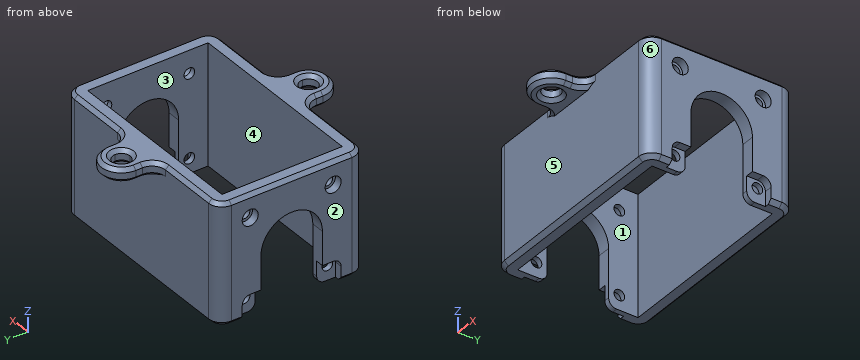
```python
from build123d import *

# Parameters (mm, degrees)
F0_W          = 70
F0_H          = 45
F1_DEPTH      = 45
F2_R          = 2
F3_DEPTH      = 40.001
F3_DEPTH_BACK = 40.001
F5_R          = 3
F6_DEPTH      = 3
F7_R          = 3
F8_DEPTH      = 3
F9_R          = 3
F10_SIZE      = 1.5
F12_DEPTH     = 5
F13_R         = 5
F14_T1_DEPTH  = 22.5
F14_T3_DEPTH  = 22.5
F14_T5_DEPTH  = 2.5
F14_T7_DEPTH  = 45
F14_T9_DEPTH  = 2.5
F14_T16_ANGLE = 180
F14_T22_ANGLE = 128.3255006626
F14_T27_ANGLE = 90
F14_T29_ANGLE = 90
F14_T31_ANGLE = 180
F14_T33_ANGLE = 90
F14_T35_ANGLE = 90
F14_T37_ANGLE = 90
F14_T39_ANGLE = 90
F14_T41_ANGLE = 180
F14_T43_ANGLE = 90
F14_T45_ANGLE = 90
F14_T49_ANGLE = 128.3255006626
F14_T52_ANGLE = 180
F14_T56_ANGLE = 128.3255006626
F14_T61_ANGLE = 128.3255006626


# Not quite as in the source:
# - a fillet or chamfer that OpenCascade refuses, or shapes differently, is made with other operations: its cross-section is extruded or revolved along the edge and cut away or added


with BuildPart() as f1:
    # F0 (on Top) → F1 (new body)
    with BuildSketch(Plane.XY):
        with BuildLine():
            ThreePointArc((40, 22.5), (38.5355339059, 26.0355339059), (35, 27.5))
            Line((35, 27.5), (-35, 27.5))
            ThreePointArc((-35, 27.5), (-38.5355339059, 26.0355339059), (-40, 22.5))
            Line((-40, 22.5), (-40, -22.5))
            ThreePointArc((-40, -22.5), (-38.5355339059, -26.0355339059), (-35, -27.5))
            Line((-35, -27.5), (35, -27.5))
            ThreePointArc((35, -27.5), (38.5355339059, -26.0355339059), (40, -22.5))
            Line((40, -22.5), (40, 22.5))
        make_face()
        Rectangle(F0_W, F0_H, mode=Mode.SUBTRACT)
    extrude(amount=F1_DEPTH)

    # F2 (on Right) → F3 (cut, two sides)
    with BuildSketch(Plane.YZ) as f3_sk:
        with Locations((15.5, 36.5)):
            Circle(F2_R)
        with Locations((-15.5, 36.5)):
            Circle(F2_R)
        with Locations((15.5, 5.5)):
            Circle(F2_R)
        with Locations((-15.5, 5.5)):
            Circle(F2_R)
        with BuildLine():
            Line((11.5, 0), (11.5, 21))
            ThreePointArc((11.5, 21), (0, 32.5), (-11.5, 21))
            Line((-11.5, 21), (-11.5, 0))
            Line((-11.5, 0), (11.5, 0))
        make_face()
    extrude(amount=-F3_DEPTH, mode=Mode.SUBTRACT)
    extrude(f3_sk.sketch, amount=F3_DEPTH_BACK, mode=Mode.SUBTRACT)

    # F5 (on face) → F6 (cut)
    with BuildSketch(Plane.YZ.offset(40)):
        with Locations((-15.5, 36.5)):
            Circle(F5_R)
        with Locations((15.5, 36.5)):
            Circle(F5_R)
        with BuildLine():
            ThreePointArc((-15.5, 8.5), (-17.6213203436, 7.6213203436), (-18.5, 5.5))
            Line((-18.5, 5.5), (-18.5, 0))
            Line((-18.5, 0), (-11.5, 0))
            Line((-11.5, 0), (-11.5, 8.5))
            Line((-11.5, 8.5), (-15.5, 8.5))
        make_face()
        with BuildLine():
            Line((15.5, 8.5), (11.5, 8.5))
            Line((11.5, 8.5), (11.5, 0))
            Line((11.5, 0), (18.5, 0))
            Line((18.5, 0), (18.5, 5.5))
            ThreePointArc((18.5, 5.5), (17.6213203436, 7.6213203436), (15.5, 8.5))
        make_face()
    extrude(amount=-F6_DEPTH, mode=Mode.SUBTRACT)

    # F7 (on face) → F8 (cut)
    with BuildSketch(Plane(origin=(-40, 0, 0), x_dir=(0, -1, 0), z_dir=(-1, 0, 0))):
        with Locations((-15.5, 36.5)):
            Circle(F7_R)
        with Locations((15.5, 36.5)):
            Circle(F7_R)
        with BuildLine():
            Line((11.5, 0), (18.5, 0))
            Line((18.5, 0), (18.5, 5.5))
            ThreePointArc((18.5, 5.5), (17.6213203436, 7.6213203436), (15.5, 8.5))
            Line((15.5, 8.5), (11.5, 8.5))
            Line((11.5, 8.5), (11.5, 0))
        make_face()
        with BuildLine():
            Line((-11.5, 8.5), (-15.5, 8.5))
            ThreePointArc((-15.5, 8.5), (-17.6213203436, 7.6213203436), (-18.5, 5.5))
            Line((-18.5, 5.5), (-18.5, 0))
            Line((-18.5, 0), (-11.5, 0))
            Line((-11.5, 0), (-11.5, 8.5))
        make_face()
    extrude(amount=-F8_DEPTH, mode=Mode.SUBTRACT)

    # F9
    f9_edges = [f1.edges().sort_by_distance(p)[0] for p in [
        (36, 11.5, 0),
        (-36, 11.5, 0),
        (-36, -11.5, 0),
        (36, -11.5, 0),
    ]]
    fillet(f9_edges, radius=F9_R)

    # F10
    f10_edges = [f1.edges().sort_by_distance(p)[0] for p in [
        (-40, 20.5, 0),
        (-38.535534, -26.035534, 0),
        (-40, -20.5, 0),
        (0, -27.5, 0),
        (38.535534, -26.035534, 0),
        (40, -20.5, 0),
        (40, 20.5, 0),
        (38.535534, 26.035534, 0),
        (0, 27.5, 0),
        (-38.535534, 26.035534, 0),
    ]]
    chamfer(f10_edges, length=F10_SIZE)

    # F11 (on face) → F12 (join)
    with BuildSketch(Plane.XY.offset(45)):
        with BuildLine():
            Line((-7.5, 27.5), (0, 27.5))
            Line((0, 27.5), (7.5, 27.5))
            Line((7.5, 27.5), (7.5, 35))
            ThreePointArc((7.5, 35), (0, 42.5), (-7.5, 35))
            Line((-7.5, 35), (-7.5, 27.5))
        make_face()
        with BuildLine():
            ThreePointArc((0, 31.75), (-2.2980970389, 37.2980970389), (3.25, 35))
            ThreePointArc((3.25, 35), (2.2980970389, 32.7019029611), (0, 31.75))
        make_face(mode=Mode.SUBTRACT)
        with BuildLine():
            Line((7.5, -22.5), (0, -22.5))
            Line((0, -22.5), (-7.5, -22.5))
            Line((-7.5, -22.5), (-7.5, -35))
            ThreePointArc((-7.5, -35), (0, -42.5), (7.5, -35))
            Line((7.5, -35), (7.5, -22.5))
        make_face()
        with BuildLine():
            ThreePointArc((3.25, -35), (-2.2980970389, -37.2980970389), (0, -31.75))
            ThreePointArc((0, -31.75), (2.2980970389, -32.7019029611), (3.25, -35))
        make_face(mode=Mode.SUBTRACT)
    extrude(amount=-F12_DEPTH)

    # F13
    f13_edges = [f1.edges().sort_by_distance(p)[0] for p in [
        (7.5, 27.5, 42.5),
        (-7.5, 27.5, 42.5),
        (-7.5, -27.5, 42.5),
        (7.5, -27.5, 42.5),
    ]]
    fillet(f13_edges, radius=F13_R)

    # F14: chamfer of 1.3 on 34 edges, made by hand

    # F14_s2 → F14_t1 (cut)
    with BuildSketch(Plane.YZ.offset(12.5)):
        Polygon((-27.5, 43.7), (-26.2, 45), (-27.5, 45), align=None)
        Polygon((26.2, 45), (27.5, 43.7), (27.5, 45), align=None)
    extrude(amount=F14_T1_DEPTH, mode=Mode.SUBTRACT)

    # F14_s4 → F14_t3 (cut)
    with BuildSketch(Plane.YZ.offset(-35)):
        Polygon((-27.5, 43.7), (-26.2, 45), (-27.5, 45), align=None)
        Polygon((26.2, 45), (27.5, 43.7), (27.5, 45), align=None)
    extrude(amount=F14_T3_DEPTH, mode=Mode.SUBTRACT)

    # F14_s6 → F14_t5 (cut)
    with BuildSketch(Plane.XZ.offset(32.5)):
        Polygon((6.2, 45), (7.5, 43.7), (7.5, 45), align=None)
        Polygon((-6.2, 45), (-7.5, 43.7), (-7.5, 45), align=None)
        Polygon((-6.2, 40), (-7.5, 41.3), (-7.5, 40), align=None)
        Polygon((6.2, 40), (7.5, 41.3), (7.5, 40), align=None)
    extrude(amount=F14_T5_DEPTH, mode=Mode.SUBTRACT)

    # F14_s8 → F14_t7 (cut)
    with BuildSketch(Plane.XZ.offset(-22.5)):
        Polygon((38.7, 45), (40, 43.7), (40, 45), align=None)
        Polygon((-38.7, 45), (-40, 43.7), (-40, 45), align=None)
    extrude(amount=F14_T7_DEPTH, mode=Mode.SUBTRACT)

    # F14_s10 → F14_t9 (cut)
    with BuildSketch(Plane.XZ.offset(-35)):
        Polygon((6.2, 45), (7.5, 43.7), (7.5, 45), align=None)
        Polygon((-6.2, 45), (-7.5, 43.7), (-7.5, 45), align=None)
        Polygon((7.5, 41.3), (6.2, 40), (7.5, 40), align=None)
        Polygon((-7.5, 41.3), (-6.2, 40), (-7.5, 40), align=None)
    extrude(amount=F14_T9_DEPTH, mode=Mode.SUBTRACT)

    # F14_s11 → F14_t12 (revolve, cut)
    with BuildSketch(Plane.XZ.offset(35)):
        Polygon((4.55, 45), (3.25, 43.7), (3.25, 45), align=None)
    revolve(axis=Axis((0, -35, 45), (0, 0, -1)), mode=Mode.SUBTRACT)

    # F14_s13 → F14_t14 (revolve, cut)
    with BuildSketch(Plane.XZ.offset(-35)):
        Polygon((4.55, 45), (3.25, 43.7), (3.25, 45), align=None)
    revolve(axis=Axis((0, 35, 45), (0, 0, -1)), mode=Mode.SUBTRACT)

    # F14_s15 → F14_t16 (revolve, cut)
    with BuildSketch(Plane.XZ.offset(-35)):
        Polygon((7.5, 41.3), (6.2, 40), (7.5, 40), align=None)
    revolve(axis=Axis((0, 35, 40), (0, 0, 1)), revolution_arc=F14_T16_ANGLE, mode=Mode.SUBTRACT)

    # F14_s17 → F14_t18 (revolve, cut)
    with BuildSketch(Plane.XZ.offset(-35)):
        Polygon((3.25, 41.3), (4.55, 40), (3.25, 40), align=None)
    revolve(axis=Axis((0, 35, 40), (0, 0, -1)), mode=Mode.SUBTRACT)


with BuildPart() as f14_tool20:
    # F14_s21 → F14_t22 (revolve)
    with BuildSketch(Plane(origin=(-23.5039658434, -18.5793051911, 0), x_dir=(0, 0, 1), z_dir=(-0.7845004474, -0.6201282512, 0))):
        Polygon((40, -11.4446614013), (41.3, -12.7446614013), (40, -12.7446614013), align=None)
    revolve(axis=Axis((-12.5, -32.5, 40), (0, 0, -1)), revolution_arc=F14_T22_ANGLE)

    split(bisect_by=Plane.XZ.offset(27.5), keep=Keep.TOP)


with BuildPart() as f1_1:
    add(f1.part)

    # F14_t19: cut F14_tool20
    add(f14_tool20.part, mode=Mode.SUBTRACT)

    # F14_s24 → F14_t25 (revolve, cut)
    with BuildSketch(Plane.XZ.offset(35)):
        Polygon((4.55, 40), (3.25, 41.3), (3.25, 40), align=None)
    revolve(axis=Axis((0, -35, 40), (0, 0, -1)), mode=Mode.SUBTRACT)

    # F14_s26 → F14_t27 (revolve, cut)
    with BuildSketch(Plane.YZ.offset(12.5)):
        Polygon((-26.2, 45), (-27.5, 43.7), (-27.5, 45), align=None)
    revolve(axis=Axis((12.5, -32.5, 45), (0, 0, 1)), revolution_arc=F14_T27_ANGLE, mode=Mode.SUBTRACT)

    # F14_s28 → F14_t29 (revolve, cut)
    with BuildSketch(Plane.YZ.offset(35)):
        Polygon((-26.2, 45), (-27.5, 43.7), (-27.5, 45), align=None)
    revolve(axis=Axis((35, -22.5, 45), (0, 0, 1)), revolution_arc=F14_T29_ANGLE, mode=Mode.SUBTRACT)

    # F14_s30 → F14_t31 (revolve, cut)
    with BuildSketch(Plane.XZ.offset(35)):
        Polygon((-6.2, 45), (-7.5, 43.7), (-7.5, 45), align=None)
    revolve(axis=Axis((0, -35, 45), (0, 0, 1)), revolution_arc=F14_T31_ANGLE, mode=Mode.SUBTRACT)

    # F14_s32 → F14_t33 (revolve, cut)
    with BuildSketch(Plane.XZ.offset(-22.5)):
        Polygon((38.7, 45), (40, 43.7), (40, 45), align=None)
    revolve(axis=Axis((35, 22.5, 45), (0, 0, 1)), revolution_arc=F14_T33_ANGLE, mode=Mode.SUBTRACT)

    # F14_s34 → F14_t35 (revolve, cut)
    with BuildSketch(Plane.YZ.offset(-12.5)):
        Polygon((-26.2, 45), (-27.5, 43.7), (-27.5, 45), align=None)
    revolve(axis=Axis((-12.5, -32.5, 45), (0, 0, -1)), revolution_arc=F14_T35_ANGLE, mode=Mode.SUBTRACT)

    # F14_s36 → F14_t37 (revolve, cut)
    with BuildSketch(Plane.YZ.offset(12.5)):
        Polygon((26.2, 45), (27.5, 43.7), (27.5, 45), align=None)
    revolve(axis=Axis((12.5, 32.5, 45), (0, 0, -1)), revolution_arc=F14_T37_ANGLE, mode=Mode.SUBTRACT)

    # F14_s38 → F14_t39 (revolve, cut)
    with BuildSketch(Plane.XZ.offset(22.5)):
        Polygon((-38.7, 45), (-40, 43.7), (-40, 45), align=None)
    revolve(axis=Axis((-35, -22.5, 45), (0, 0, 1)), revolution_arc=F14_T39_ANGLE, mode=Mode.SUBTRACT)

    # F14_s40 → F14_t41 (revolve, cut)
    with BuildSketch(Plane.XZ.offset(-35)):
        Polygon((6.2, 45), (7.5, 43.7), (7.5, 45), align=None)
    revolve(axis=Axis((0, 35, 45), (0, 0, 1)), revolution_arc=F14_T41_ANGLE, mode=Mode.SUBTRACT)

    # F14_s42 → F14_t43 (revolve, cut)
    with BuildSketch(Plane.YZ.offset(-35)):
        Polygon((26.2, 45), (27.5, 43.7), (27.5, 45), align=None)
    revolve(axis=Axis((-35, 22.5, 45), (0, 0, 1)), revolution_arc=F14_T43_ANGLE, mode=Mode.SUBTRACT)

    # F14_s44 → F14_t45 (revolve, cut)
    with BuildSketch(Plane.YZ.offset(-12.5)):
        Polygon((26.2, 45), (27.5, 43.7), (27.5, 45), align=None)
    revolve(axis=Axis((-12.5, 32.5, 45), (0, 0, 1)), revolution_arc=F14_T45_ANGLE, mode=Mode.SUBTRACT)


with BuildPart() as f14_tool47:
    # F14_s48 → F14_t49 (revolve)
    with BuildSketch(Plane(origin=(23.5039658434, -18.5793051911, 0), x_dir=(0, 0, 1), z_dir=(0.7845004474, -0.6201282512, 0))):
        Polygon((41.3, 12.7446614013), (40, 11.4446614013), (40, 12.7446614013), align=None)
    revolve(axis=Axis((12.5, -32.5, 40), (0, 0, 1)), revolution_arc=F14_T49_ANGLE)

    split(bisect_by=Plane.XZ.offset(27.5), keep=Keep.TOP)


with BuildPart() as f1_2:
    add(f1_1.part)

    # F14_t46: cut F14_tool47
    add(f14_tool47.part, mode=Mode.SUBTRACT)

    # F14_s51 → F14_t52 (revolve, cut)
    with BuildSketch(Plane.XZ.offset(35)):
        Polygon((-6.2, 40), (-7.5, 41.3), (-7.5, 40), align=None)
    revolve(axis=Axis((0, -35, 40), (0, 0, 1)), revolution_arc=F14_T52_ANGLE, mode=Mode.SUBTRACT)


with BuildPart() as f14_tool54:
    # F14_s55 → F14_t56 (revolve)
    with BuildSketch(Plane(origin=(23.5039658434, 18.5793051911, 0), x_dir=(0, 0, 1), z_dir=(0.7845004474, 0.6201282512, 0))):
        Polygon((41.3, -12.7446614013), (40, -11.4446614013), (40, -12.7446614013), align=None)
    revolve(axis=Axis((12.5, 32.5, 40), (0, 0, -1)), revolution_arc=F14_T56_ANGLE)

    split(bisect_by=Plane.XZ.offset(-27.5), keep=Keep.BOTTOM)


with BuildPart() as f1_3:
    add(f1_2.part)

    # F14_t53: cut F14_tool54
    add(f14_tool54.part, mode=Mode.SUBTRACT)


with BuildPart() as f14_tool59:
    # F14_s60 → F14_t61 (revolve)
    with BuildSketch(Plane(origin=(-23.5039658434, 18.5793051911, 0), x_dir=(0, 0, 1), z_dir=(-0.7845004474, 0.6201282512, 0))):
        Polygon((41.3, 12.7446614013), (40, 11.4446614013), (40, 12.7446614013), align=None)
    revolve(axis=Axis((-12.5, 32.5, 40), (0, 0, 1)), revolution_arc=F14_T61_ANGLE)

    split(bisect_by=Plane.XZ.offset(-27.5), keep=Keep.BOTTOM)


with BuildPart() as f1_4:
    add(f1_3.part)

    # F14_t58: cut F14_tool59
    add(f14_tool59.part, mode=Mode.SUBTRACT)


solid = f1_4.part
```
Check sheet for the modelled part. Datum: model origin and axes. Units: mm. Face numbers are marked on the shaded views. A direction names the side the tool comes from. Give positions to 0.01 mm unless a question says otherwise; leave off trailing zeros. Order: outer loops, then holes, each group sorted by start corner. A loop starts at its lowest first (then second) coordinate and runs counter-clockwise, first axis right, second up. Notation, with made-up numbers: M 73,41.5 L 100,41.5 A29 ccw 100,71.5 Z; hole C 5,42 d7. An arc over 180 degrees is marked long. Answer in a Markdown table with one row per item. Add a question column.
Q1. Thickness scan on L1, parallel to Y at x = 0, z = 43; L2, parallel to Z at x = -36.1, y = -15.5; L3, parallel to Y at x = 35.5, z = 36.5. Record the ranges inside material, lowest first.
Q2. Sectioned sample at C-C, the plane y = 0. Record the boundary of the cut face in (x, z).
Q3. Sectioned sample at A-A, the plane x = -29. Record the boundary of the cut face in (y, z), and give its area (3 significant figures).
Q4. Release check for a two-part mould opening along X. For the marked faces 3, 4, 5 and 6 record: released by +X, released by -X, zero draft, split by the parting line, or undercut.
Q5. Gauge pin test, flat ends, axial feed: pin 1 Ø5 at (x, z) = (20.5, 18) entering from +Y; pin 2 Ø0.7 at (y, z) = (-33, 42) entering from -X; pin 3 Ø4 at (x, y) = (-4, -33.5) entering from -Z; pin 4 Ø3.5 at (y, z) = (15.5, 36.5) entering from -X. Record the tip position at first contact, or that the pin passes through.
Q6. Access from +Z, -Z, +X, -X, +Y, -Y to the whole of each face (thin tool, end or side, straight path). Record for the marked faces 1 and 2.
Q7. Sectioned sample at B-B, the plane z = 12. Record the boundary of the cut face in (x, y).
Q8. Sectioned sample at D-D, the plane z = 36.5. Count the separate pieces of the cut face and the enclosed holes in it, and give its area (3 significant figures).
Verdict:
| question | item | result |
|---|---|---|
| 1 | L1 | -42.5 to -38.25, -31.75 to -22.5, 22.5 to 31.75, 38.25 to 42.5 |
| 1 | L2 | 0 to 3.5, 7.5 to 34.5, 38.5 to 45 |
| 1 | L3 | -27.47 to -17.5, -13.5 to 13.5, 17.5 to 27.47 |
| 2 | outline | M -40,32.5 L -35,32.5 L -35,45 L -38.7,45 L -40,43.7 Z; M 35,32.5 L 40,32.5 L 40,43.7 L 38.7,45 L 35,45 Z |
| 3 | outline | M -27.5,1.5 L -26,0 L -22.5,0 L -22.5,45 L -26.2,45 L -27.5,43.7 Z; M 22.5,0 L 26,0 L 27.5,1.5 L 27.5,43.7 L 26.2,45 L 22.5,45 Z |
| 3 | area | 446 mm² |
| 4 | face 3 | undercut |
| 4 | face 4 | undercut |
| 4 | face 5 | zero draft |
| 4 | face 6 | released by +X |
| 5 | pin 1 | y = 27.5 |
| 5 | pin 2 | x = -7.5 |
| 5 | pin 3 | z = 40 |
| 5 | pin 4 | through |
| 6 | face 1 | +Z, -Z |
| 6 | face 2 | +Z, -Z, -X, +Y, -Y |
| 7 | outline | M -40,-22.5 A5 ccw -35,-27.5 L 35,-27.5 A5 ccw 40,-22.5 L 40,-11.5 L 35,-11.5 L 35,-22.5 L -35,-22.5 L -35,-11.5 L -40,-11.5 Z; M -40,11.5 L -35,11.5 L -35,22.5 L 35,22.5 L 35,11.5 L 40,11.5 L 40,22.5 A5 ccw 35,27.5 L -35,27.5 A5 ccw -40,22.5 Z |
| 8 | separate pieces | 4 |
| 8 | enclosed holes | 0 |
| 8 | area | 1,120 mm² |
